Geometry: see drawing. Coordinates: mm, zero at the bounding-box minimum. Round coordinates to 2 decimals unless told otherwise and drop trailing zeros. Loops run counter-clockwise (first coordinate to the right, second up) from the corner with the lowest first, then second, coordinate; pieces in that order, holes last. Notation, with made-up numbers: (49.5, 39.5) - (72.5, 39.5) arc R7 cw to (72.5, 49.5) - close; hole circle Ø9 at (6.5, 37). An arc over 180 degrees is marked (long way). Use CSV: the item, a comma, the result in double quotes. Start each with the question number.
1. Cut plane C-C (y = 113). Return loops of the section in (x, z), and give its area (3 significant figures).
2. Cut plane A-A (z = 335). Return loops of the section in (x, y).
3. Pin query (flat end, axial travel): P1, Ø21, axis at y = 194.26, z = 58.79, coming from the +X side; P2, Ø8, axis at x = 14, z = 136, coming from the +Y side; P3, Ø3, axis at x = 20.5, y = 228.5, coming from the -Z side; P4, Ø10, axis at x = 4.5, y = 106.5, coming from the +Z side (1 decimal). Return the tip coordinate at first contact, or that it passes through.
4. Material intervals for probe 1 along Z at (x, y) = (29, 294.5) (1 decimal); probe 2 along Z at (x, y) = (27.5, 618.5) (1 decimal); probe 3 along Y at (x, z) = (10, 281.5) (1 decimal), sorted ascending. Write a range as from..to.
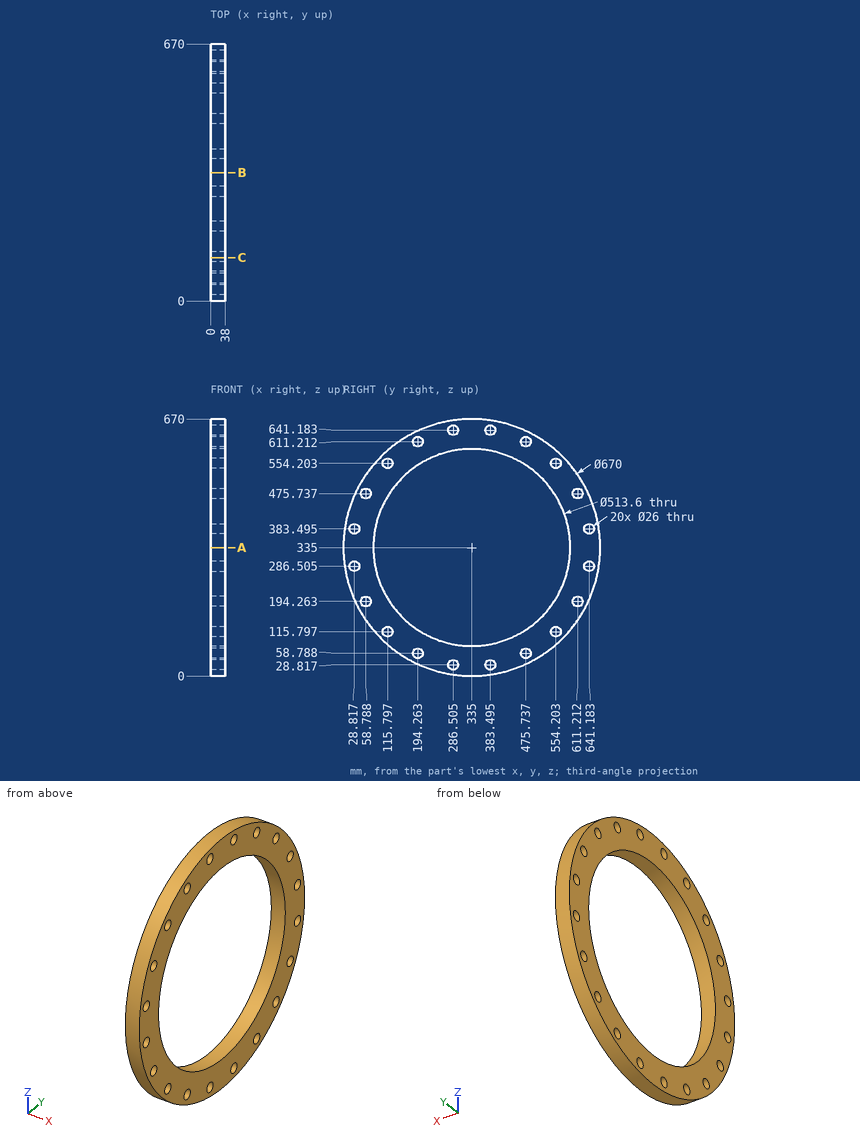
Established:
1,outline,"(0, 84.12) - (38, 84.12) - (38, 103.1) - (0, 103.1) - close; (0, 128.49) - (38, 128.49) - (38, 205.92) - (0, 205.92) - close; (0, 464.08) - (38, 464.08) - (38, 541.51) - (0, 541.51) - close; (0, 566.9) - (38, 566.9) - (38, 585.88) - (0, 585.88) - close"
1,area,"7,330 mm2"
2,outline,"(0, 0) - (38, 0) - (38, 78.2) - (0, 78.2) - close; (0, 591.8) - (38, 591.8) - (38, 670) - (0, 670) - close"
3,P1,"passes through"
3,P2,"stops at y = 607.4"
3,P3,"stops at z = 16.88"
3,P4,"stops at z = 584.5"
4,probe 1,"z = 2.5..18.6, 39.1..81.4, 588.6..630.9, 651.4..667.5"
4,probe 2,"z = 156.5..183.5, 205..465, 486.5..513.5"
4,probe 3,"y = 4.3..16.8, 40.8..83.8, 586.2..629.2, 653.2..665.7"
